Source: CAD feature listing. Evaluate the final solid. Frame: model axes, mm. Face numbers are marked on the shaded views. A direction names the side the tool comes from. Give positions to 0.01 mm unless a question says otherwise; leave off trailing zeros. Order: outer loops, then holes, each group sorted by start corner. A loop starts at its lowest first (then second) coordinate and runs counter-clockwise, first axis right, second up. Notation, with made-up numbers: M 30.5,-38.5 L 45.5,-38.5 A17 cw 45.5,-31.5 Z; hole C 58,84.25 d9. An arc over 180 degrees is marked long. Return JSON: item names as keys, results as strings.
Autodesk Inventor part; units mm, degrees
ref_plane "YZ Plane" through (0, 0, 0) normal (1, 0, 0) x (0, 1, 0)
ref_plane "XZ Plane" through (0, 0, 0) normal (0, 1, 0) x (-1, 0, 0)
ref_plane "XY Plane" through (0, 0, 0) normal (0, 0, 1) x (1, 0, 0)
sketch "Эскиз1" plane through (0, 0, 0) normal (0, 1, 0) x (-1, 0, 0)
  line L0 (0, 0) -> (0, -46)
  line L1 (0, 0) -> (10.9, 0)
  line L2 (10.9, 0) -> (10.9, -6.5)
  line L3 (10.9, -6.5) -> (9.2, -6.5)
  line L4 (9.2, -6.5) -> (9.2, -46)
  line L5 (9.2, -46) -> (0, -46)
  line L6 (0, 0) -> (-10.9, 0)
  line L7 (-10.9, 0) -> (-10.9, -6.5)
  line L8 (-10.9, -6.5) -> (-9.2, -6.5)
  line L9 (-9.2, -6.5) -> (-9.2, -46)
  line L10 (-9.2, -46) -> (0, -46)
  dimension "d1" = 6.5
  dimension "d2" = 46
  dimension "d3" = 18.4
  dimension "d4" = 21.8
extrude "Выдавливание1" add sketch "Эскиз1" along normal blind 1.5
chamfer "Фаска1" distance 2 angle 45 2 edges at (10.9, 0.75, 0) (-10.9, 0.75, 0)
chamfer "Фаска2" distance 1 angle 45 2 edges at (9.2, 0.75, -46) (-9.2, 0.75, -46)
sketch "Эскиз2" plane through (0, 1.5, 0) normal (0, 1, 0) x (1, 0, 0)
  line L0 (0, 0) -> (0, 46)
  line L1 (8.2, 46) -> (-8.2, 46)
  line L2 (-8.9, 0) -> (8.9, 0)
  point P0 (-8, 3.4)
  point P1 (8, 3.4)
  point P2 (-7, 44)
  point P3 (7, 44)
  dimension "d20" = 3.4
  dimension "d21" = 16
  dimension "d22" = 14
  dimension "d23" = 44
hole "Отверстие1" at (-8, 1.5, -3.4) at (8, 1.5, -3.4) at (-7, 1.5, -44) at (7, 1.5, -44) direction (0, -1, 0) diameter 2 end through all countersink diameter 3.2 countersink angle 90
sketch "Эскиз3" plane through (0, 0, 0) normal (0, -1, 0) x (1, 0, 0)
  line L0 (8.7, -6.9) -> (0, -6.9)
  line L1 (-8.9, 0) -> (8.9, 0)
  line L2 (8.7, -6.9) -> (8.7, -42)
  line L3 (10.9, -2) -> (10.9, -6.5)
  line L4 (8.7, -42) -> (6.2, -42)
  line L5 (4.2, -44) -> (4.2, -44)
  line L6 (4.2, -44) -> (0, -44)
  line L7 (8.7, -6.9) -> (5.8, -6.9)
  line L8 (0, 0) -> (0, -46)
  line L9 (8.2, -46) -> (-8.2, -46)
  arc A0 (6.2, -42) -> (4.2, -44) centre (6.2, -44) ccw
  line L10 (-8.7, -6.9) -> (0, -6.9)
  line L11 (-8.7, -6.9) -> (-8.7, -42)
  line L12 (-8.7, -42) -> (-6.2, -42)
  line L13 (-4.2, -44) -> (-4.2, -44)
  line L14 (-4.2, -44) -> (0, -44)
  line L15 (-8.7, -6.9) -> (-5.8, -6.9)
  arc A1 (-4.2, -44) -> (-6.2, -42) centre (-6.2, -44) ccw
  circle A2 centre (-7, -44) radius 1
  circle A3 centre (-8, -3.4) radius 1
  circle A4 centre (8, -3.4) radius 1
  circle A5 centre (7, -44) radius 1
  line L16 (-8.2, -46) -> (-9.2, -45)
  line L17 (8.2, -46) -> (-8.2, -46)
  line L18 (9.2, -45) -> (8.2, -46)
  line L19 (9.2, -6.5) -> (9.2, -45)
  line L20 (10.9, -6.5) -> (9.2, -6.5)
  line L21 (10.9, -2) -> (10.9, -6.5)
  line L22 (8.9, 0) -> (10.9, -2)
  line L23 (-8.9, 0) -> (8.9, 0)
  line L24 (-10.9, -2) -> (-8.9, 0)
  line L25 (-10.9, -6.5) -> (-10.9, -2)
  line L26 (-9.2, -6.5) -> (-10.9, -6.5)
  line L27 (-9.2, -45) -> (-9.2, -6.5)
  dimension "d24" = 6.9
  dimension "d25" = 2.2
  dimension "d26" = 42
  dimension "d27" = 44
  dimension "d28" = 6.7
  dimension "d30" = 2
extrude "Выдавливание2" add sketch "Эскиз3" along normal blind 0.8 contours L2 L4 A0 L6 L8 L0 | L8 L14 A1 L12 L11 L10
sketch "Эскиз5" plane through (0, -0.8, 0) normal (0, -1, 0) x (1, 0, 0)
  line L0 (-7.9, -42) -> (4.3, -42)
  line L1 (4.3, -42) -> (4.3, -8)
  line L2 (4.3, -8) -> (-7.9, -8)
  line L3 (-7.9, -8) -> (-7.9, -42)
  line L4 (-10.9, -6.5) -> (-10.9, -2)
  line L5 (9.2, -6.5) -> (9.2, -45)
  line L6 (-8.9, 0) -> (8.9, 0)
  line L7 (8.2, -46) -> (-8.2, -46)
  line L8 (-4.4, -42) -> (-4.4, -39)
  line L9 (-4.4, -39) -> (-7.9, -39)
  point P0 (0, 0)
  dimension "d33" = 3
  dimension "d35" = 8
  dimension "d36" = 4
  dimension "d40" = 31
  dimension "d41" = 3.5
  dimension "d55" = 12.2
extrude "Выдавливание3" cut sketch "Эскиз5" against normal blind 1.6 contours L8 L9 L3 L2 L1 L0
sketch "Эскиз6" plane through (0, 1.5, 0) normal (0, 1, 0) x (1, 0, 0)
  line L0 (-6.9, 9) -> (0.9, 9)
  line L1 (0.9, 9) -> (0.9, 35)
  line L2 (0.9, 35) -> (-6.9, 35)
  line L3 (-6.9, 35) -> (-6.9, 9)
  line L4 (-8.9, 0) -> (8.9, 0)
  line L5 (-9.2, 45) -> (-9.2, 6.5)
  line L6 (-10.9, 6.5) -> (-10.9, 2)
  line L7 (10.9, 2) -> (10.9, 6.5)
  point P0 (0, 0)
  dimension "d43" = 9
  dimension "d45" = 4
  dimension "d46" = 10
  dimension "d47" = 26
extrude "Выдавливание4" cut sketch "Эскиз6" against normal through all
fillet "Сопряжение2" radius 2 1 edges at (-0.05, 0.8, -42)
sketch "Эскиз7" plane through (0, 0, 0) normal (0, -1, 0) x (1, 0, 0)
  line L0 (-8.9, 0) -> (8.9, 0)
  line L1 (8.7, -6.9) -> (-8.7, -6.9)
  line L2 (6, 0) -> (-6, 0)
  line L3 (-6, 0) -> (-6, -6.9)
  line L4 (-6, -6.9) -> (6, -6.9)
  line L5 (6, -6.9) -> (6, 0)
  point P0 (0, 0)
  point P1 (0, 0)
  dimension "d51" = 12
extrude "Выдавливание5" add sketch "Эскиз7" along normal blind 2.8
properties part number "Case_top_new"
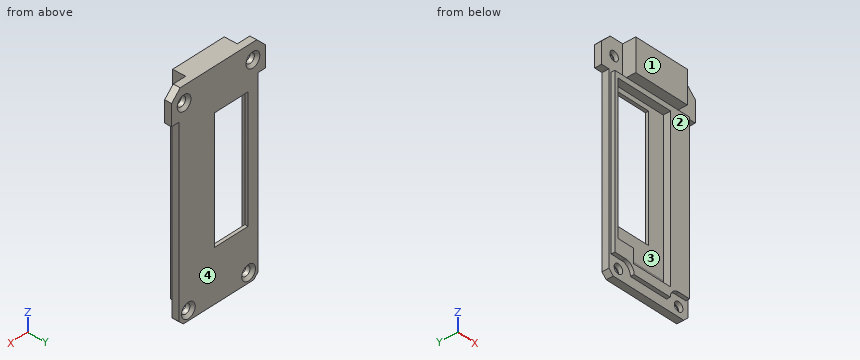
1. Section query B-B (x = 3). Return loops of the section in (y, z).
Evaluation:
{"outline": "M -2.8,-6.9 L -0.8,-6.9 L -0.8,-8 L 0.8,-8 L 0.8,-40.04 A2 cw -0.8,-42 L -0.8,-44 L 0,-44 L 0,-46 L 1.5,-46 L 1.5,0 L -2.8,0 Z"}
2. Ray query, probe 1 along X at (y, z) = (0.55, -3.4); probe 2 along X at (y, z) = (0.45, -44); probe 3 along X at (y, z) = (0.25, -27). Return the intervals inside material, ascending.
Evaluation:
{"probe 1": "x = -10.9 to -9, -7 to 7, 9 to 10.9", "probe 2": "x = -9.2 to -8, -6 to 6, 8 to 9.2", "probe 3": "x = -9.2 to -7.9, 4.3 to 9.2"}
3. Set-up query: the marked faces 1 and 2. Return all of +Z, -Z, +X, -X, +Y, -Y with unobstructed straight access to the full face (end or side cutting, diameter ignored); none if empty.
Evaluation:
{"face 1": "+Z, -Z, +X, -X, -Y", "face 2": "-Z, +X, -X, -Y"}
4. Section query A-A (z = -26.5). Return loops of the section in (x, y), then the cut area to 3 significant figures.
Evaluation:
{"outline": "M -9.2,0 L -8.7,0 L -8.7,-0.8 L -7.9,-0.8 L -7.9,0.8 L -6.9,0.8 L -6.9,1.5 L -9.2,1.5 Z; M 0.9,0.8 L 4.3,0.8 L 4.3,-0.8 L 8.7,-0.8 L 8.7,0 L 9.2,0 L 9.2,1.5 L 0.9,1.5 Z", "area": "16.5 mm^2"}
5. First-contact query: pin 1 (1.8 mm diameter, centred on y = 0, z = -41, fed in from +X); pin 2 (8.5 mm diameter, centred on x = -1.5, z = -16.5, fed in from -Y); pin 3 (5 mm diameter, centred on x = -2.5, z = -23, fed in from -Y); pin 4 (0.9 mm diameter, centred on x = -0.5, y = -0.5, fed in from -Z). Flat tips, straight axial feed; report the tip coordinate or a pass-through.
Evaluation:
{"pin 1": "stops at x = 9.2", "pin 2": "stops at y = 0.8", "pin 3": "passes through", "pin 4": "stops at z = -44"}
6. Section query C-C (z = -3.4). Return loops of the section in (x, y).
Evaluation:
{"outline": "M -10.9,0 L -9,0 L -9,0.9 L -9.6,1.5 L -10.9,1.5 Z; M -7,0 L -6,0 L -6,-2.8 L 6,-2.8 L 6,0 L 7,0 L 7,0.9 L 6.4,1.5 L -6.4,1.5 L -7,0.9 Z; M 9,0 L 10.9,0 L 10.9,1.5 L 9.6,1.5 L 9,0.9 Z"}
7. Section query D-D (y = -1.45). Return loops of the section in (x, z).
Evaluation:
{"outline": "M -6,-6.9 L 6,-6.9 L 6,0 L -6,0 Z"}
8. Draft query along X for the marked faces 3 and 4. Return one class per face: pulls with the +X half, pulls with the -X half, needs draft (parallel to the pull), parting line crosses it, or undercut.
Evaluation:
{"face 3": "undercut", "face 4": "needs draft"}
